CAD build for the part. Positions are in the model's coordinates, mm. A direction names the side the tool comes from. Give positions to 0.01 mm unless a question says otherwise; leave off trailing zeros. Order: outer loops, then holes, each group sorted by start corner. A loop starts at its lowest first (then second) coordinate and runs counter-clockwise, first axis right, second up. Notation, with made-up numbers: (-10, 15) -> (47, 15) arc R21 ccw to (47, 53) -> close; hole circle Ø9 at (26.25, 73.25). An arc over 180 degrees is marked (long way). Answer as CSV lines item,"result".
```python
from build123d import *

# Parameters (mm, degrees)
SKETCH_W        = 41
SKETCH_H        = 41
SKETCH_R        = 2
PAD_DEPTH       = 53
SKETCH001_R     = 10
SKETCH001_R_2   = 6
PAD001_DEPTH    = 1.2
FILLET_R        = 0.5
FILLET001_R     = 4
SKETCH002_W     = 3
SKETCH002_H     = 3
POCKET_DEPTH    = 2
SKETCH003_W     = 2
SKETCH003_H     = 5
POCKET001_DEPTH = 41.001
POCKET002_DEPTH = 41.001


with BuildPart() as part:
    # Sketch → Pad (new body)
    with BuildSketch(Plane.XY):
        Rectangle(SKETCH_W, SKETCH_H)
        with Locations((-16, 16)):
            Circle(SKETCH_R, mode=Mode.SUBTRACT)
        with Locations((16, 16)):
            Circle(SKETCH_R, mode=Mode.SUBTRACT)
        with Locations((-16, -16)):
            Circle(SKETCH_R, mode=Mode.SUBTRACT)
        with Locations((16, -16)):
            Circle(SKETCH_R, mode=Mode.SUBTRACT)
        with BuildLine():
            Line((-17.5, 1.2), (-7.960057, 1.2))
            ThreePointArc((-7.960057, 1.2), (-8.05, 0), (-7.960057, -1.2))
            Line((-17.5, -1.2), (-7.960057, -1.2))
            Line((-17.5, -1.2), (-17.5, -11.757359))
            ThreePointArc((-13.781771, -12.084715), (-15.605344, -11.517339), (-17.5, -11.757359))
            Line((-6.477138, -4.780082), (-13.781771, -12.084715))
            ThreePointArc((-6.477138, -4.780082), (-5.69221, -5.69221), (-4.780082, -6.477138))
            Line((-4.780082, -6.477138), (-12.084715, -13.781771))
            ThreePointArc((-11.757359, -17.5), (-11.517339, -15.605344), (-12.084715, -13.781771))
            Line((-11.757359, -17.5), (-1.2, -17.5))
            Line((-1.2, -7.960057), (-1.2, -17.5))
            ThreePointArc((-1.2, -7.960057), (0, -8.05), (1.2, -7.960057))
            Line((1.2, -7.960057), (1.2, -17.5))
            Line((1.2, -17.5), (11.757359, -17.5))
            ThreePointArc((12.084715, -13.781771), (11.517339, -15.605344), (11.757359, -17.5))
            Line((4.780082, -6.477138), (12.084715, -13.781771))
            ThreePointArc((4.780082, -6.477138), (5.69221, -5.69221), (6.477138, -4.780082))
            Line((6.477138, -4.780082), (13.781771, -12.084715))
            ThreePointArc((17.5, -11.757359), (15.605344, -11.517339), (13.781771, -12.084715))
            Line((17.5, -1.2), (17.5, -11.757359))
            Line((7.960057, -1.2), (17.5, -1.2))
            ThreePointArc((7.960057, -1.2), (8.05, 0), (7.960057, 1.2))
            Line((7.960057, 1.2), (17.5, 1.2))
            Line((17.5, 1.2), (17.5, 11.757359))
            ThreePointArc((13.781771, 12.084715), (15.605344, 11.517339), (17.5, 11.757359))
            Line((6.477138, 4.780082), (13.781771, 12.084715))
            ThreePointArc((6.477138, 4.780082), (5.69221, 5.69221), (4.780082, 6.477138))
            Line((4.780082, 6.477138), (12.084715, 13.781771))
            ThreePointArc((11.757359, 17.5), (11.517339, 15.605344), (12.084715, 13.781771))
            Line((1.2, 17.5), (11.757359, 17.5))
            Line((1.2, 7.960057), (1.2, 17.5))
            ThreePointArc((1.2, 7.960057), (0, 8.05), (-1.2, 7.960057))
            Line((-1.2, 7.960057), (-1.2, 17.5))
            Line((-11.757359, 17.5), (-1.2, 17.5))
            ThreePointArc((-12.084715, 13.781771), (-11.517339, 15.605344), (-11.757359, 17.5))
            Line((-4.780082, 6.477138), (-12.084715, 13.781771))
            ThreePointArc((-4.780082, 6.477138), (-5.69221, 5.69221), (-6.477138, 4.780082))
            Line((-6.477138, 4.780082), (-13.781771, 12.084715))
            ThreePointArc((-17.5, 11.757359), (-15.605344, 11.517339), (-13.781771, 12.084715))
            Line((-17.5, 1.2), (-17.5, 11.757359))
        make_face(mode=Mode.SUBTRACT)
    extrude(amount=PAD_DEPTH)

    # Sketch001 → Pad001 (new body)
    with BuildSketch(Plane(origin=(0, 0, 0), x_dir=(1, 0, 0), z_dir=(0, 0, -1))):
        Circle(SKETCH001_R)
        Circle(SKETCH001_R_2, mode=Mode.SUBTRACT)
    extrude(amount=-PAD001_DEPTH)

    # Fillet
    fillet_edges = [part.edges().sort_by_distance(p)[0] for p in [
        (-6.477138, 4.780082, 27.1),
        (-4.780082, 6.477138, 27.1),
        (-1.2, 7.960057, 27.1),
        (1.2, 7.960057, 27.1),
        (4.780082, 6.477138, 27.1),
        (6.477138, 4.780082, 27.1),
        (-7.960057, 1.2, 27.1),
        (-7.960057, -1.2, 27.1),
        (-6.477138, -4.780082, 27.1),
        (-4.780082, -6.477138, 27.1),
        (-1.2, -7.960057, 27.1),
        (1.2, -7.960057, 27.1),
        (4.780082, -6.477138, 27.1),
        (6.477138, -4.780082, 27.1),
        (7.960057, -1.2, 27.1),
        (7.960057, 1.2, 27.1),
    ]]
    fillet(fillet_edges, radius=FILLET_R)

    # Fillet001
    fillet001_edges = [part.edges().sort_by_distance(p)[0] for p in [
        (-20.5, 20.5, 26.5),
        (20.5, 20.5, 26.5),
        (-20.5, -20.5, 26.5),
        (20.5, -20.5, 26.5),
    ]]
    fillet(fillet001_edges, radius=FILLET001_R)

    # Sketch002 → Pocket (cut)
    with BuildSketch(Plane.XY.offset(53)):
        with Locations((6.47868, -19)):
            Rectangle(SKETCH002_W, SKETCH002_H)
    extrude(amount=-POCKET_DEPTH, mode=Mode.SUBTRACT)

    # Sketch003 → Pocket001 (cut, through all)
    with BuildSketch(Plane(origin=(0, 20.5, 0), x_dir=(-1, 0, 0), z_dir=(0, 1, 0))):
        with Locations((-10.5, 26.5)):
            Rectangle(SKETCH003_W, SKETCH003_H)
    extrude(amount=-POCKET001_DEPTH, mode=Mode.SUBTRACT)

    # Sketch004 → Pocket002 (cut, through all)
    with BuildSketch(Plane(origin=(0, 20.5, 0), x_dir=(-1, 0, 0), z_dir=(0, 1, 0))):
        Polygon((20, 29), (22, 31), (22, 22), (20, 24), align=None)
    extrude(amount=-POCKET002_DEPTH, mode=Mode.SUBTRACT)


solid = part.part
```
1) Band-saw the part on A-A, the plane y = 0. Write the cut outline in (x, z), then the cut area to 3 significant figures.
Data:
outline,"(-20.5, 0) -> (-6, 0) -> (-6, 1.2) -> (-8.05, 1.2) -> (-8.05, 53) -> (-20.5, 53) -> (-20.5, 29.5) -> (-20, 29) -> (-20, 24) -> (-20.5, 23.5) -> close; (6, 0) -> (20.5, 0) -> (20.5, 53) -> (8.05, 53) -> (8.05, 1.2) -> (6, 1.2) -> close; hole (9.5, 24) -> (11.5, 24) -> (11.5, 29) -> (9.5, 29) -> close"
area,"1,310 mm2"
2) Pull direction X, two halves, no side cores. Call faces 6 (the flat face through (13, 1.2, 26)), 7 (the flat face through (0, 20.5, 26)): pulls with the +X half, pulls with the -X half, needs draft (parallel to the pull), parting line crosses it, or undercut.
Data:
face 6,"undercut"
face 7,"needs draft"
3) Band-saw the part on C-C, the plane z = 13. Give the number of separate pieces and of enclosed holes in the cut face, then the cut area to 3 significant figures.
Data:
separate pieces,"1"
enclosed holes,"5"
area,"705 mm2"
4) Which spindle directions (+Z, -Z, +X, -X, +Y, -Y) get a long thin tool onto all of the face, cutting with end or side? Do faces 1 (the flat face through (4.979, -19, 52)), 2 (the flat face through (0, -20.5, 26)), 3 (the cylindrical face through (9.224, 3.862, 0.592)), 4 (the cylindrical face through (8.05, -0.01, 26.74)), 5 (the flat face through (11, 11, 24)). Say none if no direction does.
Data:
face 1,"+Z, -Y"
face 2,"+Z, -Z, +X, -X, -Y"
face 3,"+Z, -Z"
face 4,"+Z"
face 5,"+Y, -Y"
5) Pin check, flat tips, straight feed: P1, Ø1.5, axis at y = 18.5, z = 27.5, coming from the -X side; P2, Ø3.5, axis at y = 19.5, z = 27, coming from the +X side. Stop position of each tip, or through.
Data:
P1,"stops at x = -20"
P2,"stops at x = 20.3"
6) Band-saw the part on B-B, the plane x = 0. Write the cut outline in (y, z), then the cut area to 3 significant figures.
Data:
outline,"(-20.5, 0) -> (-6, 0) -> (-6, 1.2) -> (-8.05, 1.2) -> (-8.05, 53) -> (-20.5, 53) -> close; (6, 0) -> (20.5, 0) -> (20.5, 53) -> (8.05, 53) -> (8.05, 1.2) -> (6, 1.2) -> close"
area,"1,320 mm2"
7) Wall check: line 1 along Y through (x, z) = (16, 41); line 2 along Y through (x, z) = (15.5, 33); line 3 along X through (y, z) = (17, 5.5). Give the ranges that are in metal, low to high. Write a range as [from, to].
Data:
line 1,"y = [-20.5, -18], [-14, -11.5], [-1.2, 1.2], [11.5, 14], [18, 20.5]"
line 2,"y = [-20.5, -17.94], [-14.06, -11.53], [-1.2, 1.2], [11.53, 14.06], [17.94, 20.5]"
line 3,"x = [-20.47, -17.73], [-14.27, -11.61], [-1.2, 1.2], [11.61, 14.27], [17.73, 20.47]"
